Input: part model. Units: mm. Frame: model coordinates. A direction names the side the tool comes from. Coordinates: 2 decimals unless noted, no trailing zeros. Loops run counter-clockwise (first coordinate to the right, second up) from the corner with the lowest first, then second, coordinate; pieces in that order, holes last. Notation, with made-up numbers: (71.5, 55.25) -> (92.5, 55.25) arc R15 ccw to (92.5, 84.25) -> close; hole circle Ø5 at (35, 34.25). An arc over 180 degrees is marked (long way). Answer as a JSON object with one key per item and string values.
from build123d import *

# Parameters (mm, degrees)
BOSS_EXTRUDE1_DEPTH = 5
CUT_EXTRUDE1_DEPTH  = 52.53882032
SKETCH4_W           = 70
SKETCH4_H           = 5
BOSS_EXTRUDE2_DEPTH = 30
SKETCH5_R           = 2.5
CUT_EXTRUDE2_DEPTH  = 30
FILLET1_START       = -36
FILLET1_DEPTH       = 72
FILLET1_START_2     = -35
FILLET1_2_DEPTH     = 70


with BuildPart() as part:
    # Sketch2 → Boss-Extrude1 (new body)
    with BuildSketch(Plane.XY):
        with BuildLine():
            Line((-30, -37.5), (30, -37.5))
            ThreePointArc((30, -37.5), (33.535533906, -36.035533906), (35, -32.5))
            Line((35, -32.5), (35, 37.5))
            Line((35, 37.5), (-35, 37.5))
            Line((-35, 37.5), (-35, -32.5))
            ThreePointArc((-35, -32.5), (-33.535533906, -36.035533906), (-30, -37.5))
        make_face()
    extrude(amount=BOSS_EXTRUDE1_DEPTH)

    # Sketch3 → Cut-Extrude1 (cut, through all)
    with BuildSketch(Plane.XY.offset(5)):
        with BuildLine():
            Line((-21, 24), (-21, 16))
            ThreePointArc((-21, 16), (-23.5, 13.5), (-26, 16))
            Line((-26, 16), (-26, 24))
            ThreePointArc((-26, 24), (-23.5, 26.5), (-21, 24))
        make_face()
        with BuildLine():
            Line((-21, -23), (-21, -31))
            ThreePointArc((-21, -31), (-23.5, -33.5), (-26, -31))
            Line((-26, -31), (-26, -23))
            ThreePointArc((-26, -23), (-23.5, -20.5), (-21, -23))
        make_face()
        with BuildLine():
            Line((26, 24), (26, 16))
            ThreePointArc((26, 16), (23.5, 13.5), (21, 16))
            Line((21, 16), (21, 24))
            ThreePointArc((21, 24), (23.5, 26.5), (26, 24))
        make_face()
        with BuildLine():
            Line((26, -23), (26, -31))
            ThreePointArc((26, -31), (23.5, -33.5), (21, -31))
            Line((21, -31), (21, -23))
            ThreePointArc((21, -23), (23.5, -20.5), (26, -23))
        make_face()
        with BuildLine():
            Line((20, 0.5), (20, -7.5))
            ThreePointArc((20, -7.5), (0, -27.5), (-20, -7.5))
            Line((-20, -7.5), (-20, 0.5))
            ThreePointArc((-20, 0.5), (0, 20.5), (20, 0.5))
        make_face()
    extrude(amount=-CUT_EXTRUDE1_DEPTH, mode=Mode.SUBTRACT)

    # Sketch4 → Boss-Extrude2 (add)
    with BuildSketch(Plane.XY.offset(5)):
        with Locations((0, 35)):
            Rectangle(SKETCH4_W, SKETCH4_H)
    extrude(amount=BOSS_EXTRUDE2_DEPTH)

    # Sketch5 → Cut-Extrude2 (cut)
    with BuildSketch(Plane.XZ.offset(-32.5)):
        with Locations(Location((-12.5, 12.5, 0), (0, 0, 270))):
            Circle(SKETCH5_R)
        with Locations(Location((12.5, 12.5, 0), (0, 0, 270))):
            Circle(SKETCH5_R)
        with Locations(Location((-25, 27.5, 0), (0, 0, 270))):
            Circle(SKETCH5_R)
        with Locations(Location((25, 27.5, 0), (0, 0, 270))):
            Circle(SKETCH5_R)
    extrude(amount=-CUT_EXTRUDE2_DEPTH, mode=Mode.SUBTRACT)

    # Fillet1: read off the stored shape, not the designer's step
    # Fillet1 outline → Fillet1 (cut)
    with BuildSketch(Plane.YZ.offset(FILLET1_START)):
        with BuildLine():
            ThreePointArc((37.5, 5), (36.035533906, 1.464466094), (32.5, 0))
            Line((32.5, 0), (37.5, 0))
            Line((37.5, 0), (37.5, 5))
        make_face()
    extrude(amount=FILLET1_DEPTH, mode=Mode.SUBTRACT)

    # Fillet1 2 outline → Fillet1 2 (add)
    with BuildSketch(Plane.YZ.offset(FILLET1_START_2)):
        with BuildLine():
            Line((32.5, 5), (32.5, 10))
            ThreePointArc((32.5, 10), (31.035533906, 6.464466094), (27.5, 5))
            Line((27.5, 5), (32.5, 5))
        make_face()
    extrude(amount=FILLET1_2_DEPTH)


solid = part.part
1. Section query B-B (x = 0). Return loops of the section in (y, z), plus the area to 3 significant figures.
Reply:
{"outline": "(-37.5, 0) -> (-27.5, 0) -> (-27.5, 5) -> (-37.5, 5) -> close; (20.5, 0) -> (32.5, 0) arc R5 ccw to (37.5, 5) -> (37.5, 35) -> (32.5, 35) -> (32.5, 10) arc R5 cw to (27.5, 5) -> (20.5, 5) -> close", "area": "285 mm2"}
2. Pin query (flat end, axial travel): P1, Ø1, axis at x = 22, y = 24, coming from the -Z side; P2, Ø3, axis at x = 20.5, z = 7.5, coming from the -Y side; P3, Ø8, axis at x = -25, z = 27.5, coming from the +Y side; P4, Ø6.5, axis at x = 25, z = 27.5, coming from the -Y side. Return the tip coordinate at first contact, or that it passes through.
Reply:
{"P1": "passes through", "P2": "stops at y = 30.5", "P3": "stops at y = 37.5", "P4": "stops at y = 32.5"}
3. Line query: line 1 along X through (y, z) = (34.6, 27.5); line 2 along X through (y, z) = (36.35, 12.5); line 3 along Z through (x, y) = (-21.5, 26). Output: solid intervals per line, ascending.
Reply:
{"line 1": "x = -35 to -27.5, -22.5 to 22.5, 27.5 to 35", "line 2": "x = -35 to -15, -10 to 10, 15 to 35", "line 3": "z = 0 to 5"}
4. Section query A-A (z = 12.5). Return loops of the section in (x, y), plus the area to 3 significant figures.
Reply:
{"outline": "(-35, 32.5) -> (-15, 32.5) -> (-15, 37.5) -> (-35, 37.5) -> close; (-10, 32.5) -> (10, 32.5) -> (10, 37.5) -> (-10, 37.5) -> close; (15, 32.5) -> (35, 32.5) -> (35, 37.5) -> (15, 37.5) -> close", "area": "300 mm2"}
5. Section query D-D (x = 11). Return loops of the section in (y, z), plus the area to 3 significant figures.
Reply:
{"outline": "(-37.5, 0) -> (-24.2, 0) -> (-24.2, 5) -> (-37.5, 5) -> close; (17.2, 0) -> (32.5, 0) arc R5 ccw to (37.5, 5) -> (37.5, 10.5) -> (32.5, 10.5) -> (32.5, 10) arc R5 cw to (27.5, 5) -> (17.2, 5) -> close; (32.5, 14.5) -> (37.5, 14.5) -> (37.5, 35) -> (32.5, 35) -> close", "area": "298 mm2"}
6. Mould query, pull axis Y, two halves, no side actions, for faces 4 (the face through (-0.49, 36.07, 1.5)), 5 (the face through (-23.4, 13.5, 2.5)), 6 (the face through (27.48, 34.97, 27.83)), 7 (the face through (33.5, -36.07, 2.46)). Classes: pulls with the +Y half, pulls with the -Y half, needs draft (parallel to the pull), parting line crosses it, or undercut.
Reply:
{"face 4": "pulls with the +Y half", "face 5": "undercut", "face 6": "needs draft", "face 7": "pulls with the -Y half"}
7. Section query C-C (y = 7). Return loops of the section in (x, z), plus the area to 3 significant figures.
Reply:
{"outline": "(-35, 0) -> (-18.91, 0) -> (-18.91, 5) -> (-35, 5) -> close; (18.91, 0) -> (35, 0) -> (35, 5) -> (18.91, 5) -> close", "area": "161 mm2"}
8. Access query for faces 1 (the face through (-26, -27, 3)), 2 (the face through (0, -37.5, 2)), 3 (the face through (0, 32.5, 22)). Directions: +Z, -Z, +X, -X, +Y, -Y. A direction counts if a zero-diameter tool reaches every point of the face in a straight line with its end or side. Return the directions, or none.
Reply:
{"face 1": "+Z, -Z", "face 2": "+Z, -Z, +X, -X, -Y", "face 3": "+Z, +X, -X, -Y"}
